```python
from build123d import *

# Parameters (mm, degrees)
SKETCH_1_R      = 1.65
EXTRUDE_1_DEPTH = 2.5


with BuildPart() as part:
    # 草图1 → 凸台-拉伸1 (new body)
    with BuildSketch(Plane(origin=(0, 0, 0), x_dir=(1, 0, 0), z_dir=(0, 1, 0))):
        Polygon((85.273637, -129.294264731), (135.120165849, -129.294264731), (135.120165849, 130.705735269), (85.273637, 130.705735269), (43.120165849, 130.705735269), (43.120165849, 123.705735269), (31.120165849, 17.705735269), (31.120165849, -16.294264731), (43.120165849, -122.294264731), (43.120165849, -129.294264731), align=None)
        with Locations(Location((105.120165849, 70.205735269, 0), (0, 0, 270))):
            Circle(SKETCH_1_R, mode=Mode.SUBTRACT)
        with Locations(Location((75.120165849, 70.205735269, 0), (0, 0, 270))):
            Circle(SKETCH_1_R, mode=Mode.SUBTRACT)
        with Locations(Location((75.120165849, -68.794264731, 0), (0, 0, 90))):
            Circle(SKETCH_1_R, mode=Mode.SUBTRACT)
        with Locations(Location((105.120165849, -68.794264731, 0), (0, 0, 90))):
            Circle(SKETCH_1_R, mode=Mode.SUBTRACT)
        with Locations(Location((129.120165849, 40.705735269, 0), (0, 0, 270))):
            Circle(SKETCH_1_R, mode=Mode.SUBTRACT)
        with Locations(Location((129.120165849, -39.294264731, 0), (0, 0, 90))):
            Circle(SKETCH_1_R, mode=Mode.SUBTRACT)
    extrude(amount=EXTRUDE_1_DEPTH)


solid = part.part
```
Design review of the part built by this model. Coordinates are the model's own, in mm. Coordinates: 2 decimals unless noted, no trailing zeros. Write each loop counter-clockwise with the first axis right and the second up, starting at its lowest first coordinate (ties: lowest second). Pieces come first, ordered by that corner, then holes.
1) Insertion check: pin 1 (0.8 mm diameter, centred on y = 1, z = 126.5, fed in from -X). The pin has a flat end and moves straight along its axis. Give the tip position at first contact, or say it passes through.
2) Add section A-A (y = 0.8). Write out the cut boundary in (x, z), plus the area to 3 significant figures.
3) To check wall thickness, follow L1, parallel to X at y = 1.9, z = -71; L2, parallel to X at y = 0.5, z = -99; L3, parallel to X at y = 1.9, z = 100. State the ranges of each line that lie inside material, in increasing order.
4) Add section C-C (z = 34). Write out the cut boundary in (x, y), plus the area to 3 significant figures.
5) Add section B-B (z = -50). Write out the cut boundary in (x, y).
Check result:
1. pin 1: stops at x = 43.12
2. outline: (31.12, -17.71) - (43.12, -123.71) - (43.12, -130.71) - (135.12, -130.71) - (135.12, 129.29) - (43.12, 129.29) - (43.12, 122.29) - (31.12, 16.29) - close; hole circle Ø3.3 at (75.12, -70.21); hole circle Ø3.3 at (75.12, 68.79); hole circle Ø3.3 at (105.12, -70.21); hole circle Ø3.3 at (105.12, 68.79); hole circle Ø3.3 at (129.12, -40.71); hole circle Ø3.3 at (129.12, 39.29)
2. area: 25,500 mm2
3. L1: x = 37.15 to 73.67, 76.57 to 103.67, 106.57 to 135.12
3. L2: x = 40.32 to 135.12
3. L3: x = 40.6 to 135.12
4. outline: (33.12, 0) - (135.12, 0) - (135.12, 2.5) - (33.12, 2.5) - close
4. area: 255 mm2
5. outline: (34.78, 0) - (135.12, 0) - (135.12, 2.5) - (34.78, 2.5) - close
